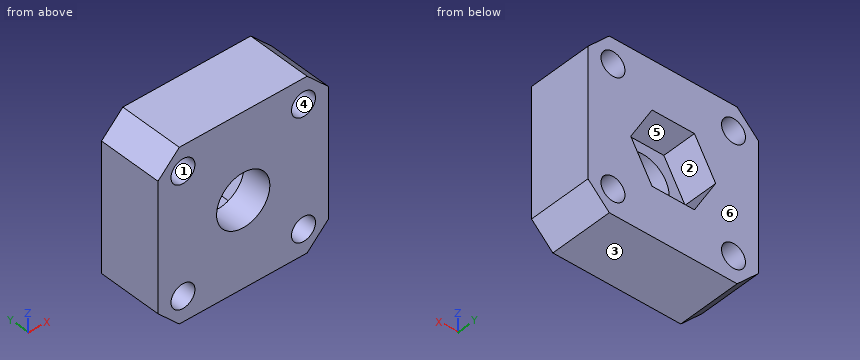
from build123d import *

# Parameters (mm, degrees)
SKETCH1_W           = 32
SKETCH1_H           = 32
SKETCH1_R           = 5
SKETCH1_R_2         = 2.25
BOSS_EXTRUDE1_DEPTH = 12
CHAMFER1_SIZE       = 4
CUT_EXTRUDE1_DEPTH  = 6.5


with BuildPart() as part:
    # Sketch1 → Boss-Extrude1 (new body)
    with BuildSketch(Plane(origin=(0, 0, 0), x_dir=(1, 0, 0), z_dir=(0, 1, 0))):
        Rectangle(SKETCH1_W, SKETCH1_H)
        with Locations(Location((0, 0, 0), (0, 0, 270))):
            Circle(SKETCH1_R, mode=Mode.SUBTRACT)
        with Locations(Location((-11.313708499, 11.313708499, 0), (0, 0, 270))):
            Circle(SKETCH1_R_2, mode=Mode.SUBTRACT)
        with Locations(Location((-11.313708499, -11.313708499, 0), (0, 0, 270))):
            Circle(SKETCH1_R_2, mode=Mode.SUBTRACT)
        with Locations(Location((11.313708499, -11.313708499, 0), (0, 0, 270))):
            Circle(SKETCH1_R_2, mode=Mode.SUBTRACT)
        with Locations(Location((11.313708499, 11.313708499, 0), (0, 0, 270))):
            Circle(SKETCH1_R_2, mode=Mode.SUBTRACT)
    extrude(amount=BOSS_EXTRUDE1_DEPTH)

    # Chamfer1
    chamfer1_edges = [part.edges().sort_by_distance(p)[0] for p in [
        (16, 6, 16),
        (-16, 6, 16),
        (-16, 6, -16),
        (16, 6, -16),
    ]]
    chamfer(chamfer1_edges, length=CHAMFER1_SIZE)

    # Sketch4 → Cut-Extrude1 (cut)
    with BuildSketch(Plane(origin=(0, 12, 0), x_dir=(1, 0, 0), z_dir=(0, 1, 0))):
        Polygon((3.983716857, -6.9), (7.967433715, 0), (3.983716857, 6.9), (-3.983716857, 6.9), (-7.967433715, 0), (-3.983716857, -6.9), align=None)
    extrude(amount=-CUT_EXTRUDE1_DEPTH, mode=Mode.SUBTRACT)


solid = part.part
Read the model definition and answer for the solid it produces. Units are mm, in the model's axes. Face numbers are marked on the shaded views. A direction names the side the tool comes from. Give positions to 0.01 mm unless a question says otherwise; leave off trailing zeros. Write each loop counter-clockwise with the first axis right and the second up, starting at its lowest first coordinate (ties: lowest second). Pieces come first, ordered by that corner, then holes. Notation, with made-up numbers: (-25.5, -26) -> (6.5, -26) arc R25 cw to (6.5, 9) -> close; hole circle Ø11 at (-26.75, 71.5). An arc over 180 degrees is marked (long way). Answer as a JSON object with one key per item and string values. Group by question number.
1) The mould has two halves that part along Z. Classify the marked faces 3, 4, 5 and 6: +Z half, -Z half, draft (parallel to the pull), parting line (faces both ways), or undercut.
2) Each of these flat-tipped pins is pushed along its axis until it touches: P1, Ø5, axis at x = -11.31, z = 11.31, coming from the +Y side; P2, Ø4, axis at x = 11.31, z = -11.31, coming from the +Y side; P3, Ø4, axis at x = 4, z = 0, coming from the +Y side. Where does it stop, or does it pass through?
3) Find section A-A (x = 0). Write down the section's boundary in (y, z).
4) Find section C-C (z = 11). Write down the section's boundary in (x, y), and give its area (3 significant figures).
5) Consider L1, parallel to X at y = 4.15, z = 0; L2, parallel to Z at x = -13, y = 9.25. Determine where each line is inside the solid, lowest interval first. Write a range as from..to.
6) A tool of negligible diameter and unlimited length cuts with its end or side. For the marked faces 1 and 2, from which of +Z, -Z, +X, -X, +Y, -Y can it reach the whole face along a straight path? Write none if from no direction.
7) Find section D-D (z = -4). Write down the section's boundary in (x, y), and give its area (3 significant figures).
8) Find section B-B (y = 2). Write down the section's boundary in (x, z).
Values follow:
{
 "1": {"face 3": "-Z half", "face 4": "undercut", "face 5": "undercut", "face 6": "draft"},
 "2": {"P1": "stops at y = 12", "P2": "passes through", "P3": "stops at y = 5.5"},
 "3": {"outline": "(0, -16) -> (12, -16) -> (12, -6.9) -> (5.5, -6.9) -> (5.5, -5) -> (0, -5) -> close; (0, 5) -> (5.5, 5) -> (5.5, 6.9) -> (12, 6.9) -> (12, 16) -> (0, 16) -> close"},
 "4": {"outline": "(-16, 0) -> (-13.54, 0) -> (-13.54, 12) -> (-16, 12) -> close; (-9.09, 0) -> (9.09, 0) -> (9.09, 12) -> (-9.09, 12) -> close; (13.54, 0) -> (16, 0) -> (16, 12) -> (13.54, 12) -> close", "area": "277 mm2"},
 "5": {"L1": "x = -16..-5, 5..16", "L2": "z = -15..-12.8, -9.82..9.82, 12.8..15"},
 "6": {"face 1": "+Y, -Y", "face 2": "+Y"},
 "7": {"outline": "(-16, 0) -> (-3, 0) -> (-3, 5.5) -> (-5.66, 5.5) -> (-5.66, 12) -> (-16, 12) -> close; (3, 0) -> (16, 0) -> (16, 12) -> (5.66, 12) -> (5.66, 5.5) -> (3, 5.5) -> close", "area": "277 mm2"},
 "8": {"outline": "(-16, -12) -> (-12, -16) -> (12, -16) -> (16, -12) -> (16, 12) -> (12, 16) -> (-12, 16) -> (-16, 12) -> close; hole circle Ø4.5 at (-11.31, -11.31); hole circle Ø4.5 at (-11.31, 11.31); hole circle Ø10 at (0, 0); hole circle Ø4.5 at (11.31, -11.31); hole circle Ø4.5 at (11.31, 11.31)"}
}
